Verification items for the finished model (mm, model axes). Coordinates: 2 decimals unless noted, no trailing zeros. Order: outer loops, then holes, each group sorted by start corner. A loop starts at its lowest first (then second) coordinate and runs counter-clockwise, first axis right, second up. Notation, with made-up numbers: (22, -17.5) -> (43, -17.5) arc R33 ccw to (43, 11.5) -> close; hole circle Ø2 at (26, 14.5). An arc over 180 degrees is marked (long way). Answer as CSV lines item,"result".
```python
from build123d import *

# Parameters (mm, degrees)
SKETCH1_W                = 232.41
SKETCH1_H                = 163.2712
BOSS_EXTRUDE1_DEPTH      = 3.175
SKETCH2_W                = 82.55
SKETCH2_H                = 21.209
CUT_EXTRUDE1_DEPTH       = 143.049476723
FILLET1_R                = 3.175
LPATTERN1_COUNT          = 2
LPATTERN1_PITCH          = 104.9866582
FILLET1_OF_LPATTERN1_R   = 3.175
CUT_EXTRUDE4_START       = -3.175
CUT_EXTRUDE4_OUTLINE_R   = 5.92074
CUT_EXTRUDE4_OUTLINE_W   = 163.40074
CUT_EXTRUDE4_OUTLINE_H   = 30.8991
CUT_EXTRUDE4_OUTLINE_R_2 = 1.75
CUT_EXTRUDE4_DEPTH       = 3.175


# Read off the part's stored shape, not the designer's step: Cut-Extrude4
with BuildPart() as part:
    # Sketch1 → Boss-Extrude1 (new body)
    with BuildSketch(Plane(origin=(0, 0, 0), x_dir=(1, 0, 0), z_dir=(0, 1, 0))):
        Rectangle(SKETCH1_W, SKETCH1_H)
    extrude(amount=-BOSS_EXTRUDE1_DEPTH)

    # Sketch2 → Cut-Extrude1 (cut, through all)
    with BuildSketch(Plane(origin=(0, 0, 0), x_dir=(1, 0, 0), z_dir=(0, 1, 0))):
        with Locations((-52.49333418, 45.6311)):
            Rectangle(SKETCH2_W, SKETCH2_H)
    cut_extrude1 = extrude(amount=-CUT_EXTRUDE1_DEPTH, mode=Mode.SUBTRACT)

    # Fillet1
    fillet1_edges = [part.edges().sort_by_distance(p)[0] for p in [
        (-93.76833418, -1.5875, -35.0266),
        (-93.76833418, -1.5875, -56.2356),
        (-11.21833418, -1.5875, -56.2356),
        (-11.21833418, -1.5875, -35.0266),
    ]]
    fillet(fillet1_edges, radius=FILLET1_R)

    # LPattern1: Cut-Extrude1 ×2
    with Locations(*[(i * LPATTERN1_PITCH, 0, 0) for i in range(1, LPATTERN1_COUNT)]):
        add(cut_extrude1, mode=Mode.SUBTRACT)

    # Fillet1 of LPattern1
    fillet1_of_lpattern1_edges = [part.edges().sort_by_distance(p)[0] for p in [
        (11.21832402, -1.5875, -35.0266),
        (11.21832402, -1.5875, -56.2356),
        (93.76832402, -1.5875, -56.2356),
        (93.76832402, -1.5875, -35.0266),
    ]]
    fillet(fillet1_of_lpattern1_edges, radius=FILLET1_OF_LPATTERN1_R)

    # Cut-Extrude4 outline → Cut-Extrude4 (cut)
    with BuildSketch(Plane(origin=(0, 0, 0), x_dir=(1, 0, 0), z_dir=(0, 1, 0)).offset(CUT_EXTRUDE4_START)):
        with Locations((-64.529208, -15.98168)):
            Circle(CUT_EXTRUDE4_OUTLINE_R)
        with Locations((-46.091348, -15.98168)):
            Circle(CUT_EXTRUDE4_OUTLINE_R)
        with Locations((-27.653488, -15.98168)):
            Circle(CUT_EXTRUDE4_OUTLINE_R)
        with Locations((-9.215628, -15.98168)):
            Circle(CUT_EXTRUDE4_OUTLINE_R)
        with Locations((9.222232, -15.98168)):
            Circle(CUT_EXTRUDE4_OUTLINE_R)
        with Locations((27.660092, -15.98168)):
            Circle(CUT_EXTRUDE4_OUTLINE_R)
        with Locations((46.097952, -15.98168)):
            Circle(CUT_EXTRUDE4_OUTLINE_R)
        with Locations((64.535812, -15.98168)):
            Circle(CUT_EXTRUDE4_OUTLINE_R)
        with Locations((0, 12.16787)):
            Rectangle(CUT_EXTRUDE4_OUTLINE_W, CUT_EXTRUDE4_OUTLINE_H)
        with Locations((-90, 25.41778)):
            Circle(CUT_EXTRUDE4_OUTLINE_R_2)
        with Locations((-90, -1.08222)):
            Circle(CUT_EXTRUDE4_OUTLINE_R_2)
        with Locations((85, -1.08222)):
            Circle(CUT_EXTRUDE4_OUTLINE_R_2)
        with Locations((85, 25.41778)):
            Circle(CUT_EXTRUDE4_OUTLINE_R_2)
    extrude(amount=CUT_EXTRUDE4_DEPTH, mode=Mode.SUBTRACT)


solid = part.part
```
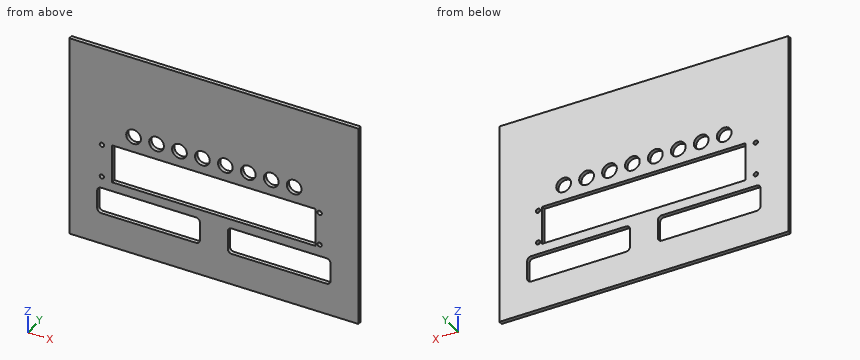
Item 1: Thickness scan on line 1 (Z direction, x = 85, y = -1.7); line 2 (Z direction, x = -56.5, y = -2.2); line 3 (X direction, y = -1.4, z = 1.5) (3 decimals). Record the ranges inside material, lowest first.
Answer list:
line 1,"-81.64 to -56.24, -35.03 to -27.17, -23.67 to -0.67, 2.83 to 81.64"
line 2,"-81.64 to -56.24, -35.03 to -27.62, 3.28 to 81.64"
line 3,"-116.205 to -91.699, -88.301 to -81.7, 81.7 to 83.301, 86.699 to 116.205"
Item 2: Section check C-C, the plane y = -1.15. Count the separate pieces of the cut face and the enclosed holes in it, plus the area to 3 significant figures.
Answer list:
separate pieces,"1"
enclosed holes,"15"
area,"28,500 mm2"
Item 3: Depth check by flat-ended pin: pin 1 Ø7 at (x, z) = (-64.53, 15.98) entering from -Y. Enter the tip coordinate at first touch or a pass-through.
Answer list:
pin 1,"through"
Item 4: Section check B-B, the plane x = 61.5. Record the boundary of the cut face in (y, z) (3 decimals), plus the area to 3 significant figures.
Answer list:
outline,"(-3.175, -81.636) -> (0, -81.636) -> (0, -56.236) -> (-3.175, -56.236) -> close; (-3.175, -35.027) -> (0, -35.027) -> (0, -27.617) -> (-3.175, -27.617) -> close; (-3.175, 3.282) -> (0, 3.282) -> (0, 10.898) -> (-3.175, 10.898) -> close; (-3.175, 21.065) -> (0, 21.065) -> (0, 81.636) -> (-3.175, 81.636) -> close"
area,"321 mm2"
Item 5: Section check A-A, the plane x = -17.5. Record the boundary of the cut face in (y, z) (3 decimals).
Answer list:
outline,"(-3.175, -81.636) -> (0, -81.636) -> (0, -56.236) -> (-3.175, -56.236) -> close; (-3.175, -35.027) -> (0, -35.027) -> (0, -27.617) -> (-3.175, -27.617) -> close; (-3.175, 3.282) -> (0, 3.282) -> (0, 81.636) -> (-3.175, 81.636) -> close"
